The listing builds one solid part. Answer for the finished solid, in the listing's coordinates (mm). Face numbers are marked on the shaded views. Coordinates: 2 decimals unless noted, no trailing zeros. Order: outer loops, then holes, each group sorted by start corner. A loop starts at its lowest first (then second) coordinate and runs counter-clockwise, first axis right, second up. Notation, with made-up numbers: M 10,30.25 L 31,30.25 A15 ccw 31,45.25 Z; hole C 52,59.5 d9. An arc over 180 degrees is marked long. One line per item, written item: value. Start each with the question number.
Q1. Each of these flat-tipped pins is pushed along its axis until it touches: pin 1 Ø5 at (x, z) = (-2, 1) entering from -Y; pin 2 Ø2 at (x, y) = (3, 2) entering from -Z; pin 3 Ø4 at (x, z) = (-3.5, 3.5) entering from +Y; pin 4 Ø5 at (x, y) = (3, -3.5) entering from -Z. Where does it stop, or does it pass through?
Q2. Straight lines are drawn through the part: line 1 along Z through (x, y) = (0, -2); line 2 along X through (y, z) = (1.25, 2); line 3 along X through (y, z) = (-1, -0.5). For each, find the intervals that lie inside material, in ascending order. Write a range as [from, to].
Q3. The part is cut by section B-B on z = 0. Give the vertices of the cut face in (x, y), then the cut area to 3 significant figures.
Q4. Determine the mould class of the marked faces 1 and 2 for opening direction Z: pulls with the +Z half, pulls with the -Z half, needs draft (parallel to the pull), parting line crosses it, or undercut.
Q5. The part is cut by section A-A on x = 0. Give the vertices of the cut face in (y, z).
Q6. The part is cut by section C-C on y = 4. Give the vertices of the cut face in (x, z).
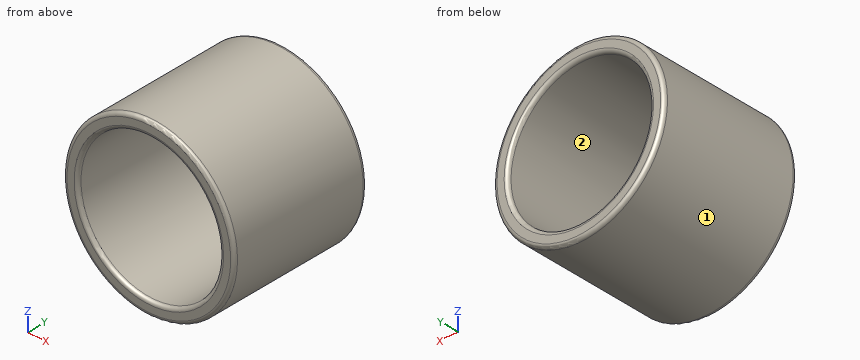
```python
from build123d import *

# Parameters (mm, degrees)
F0_R     = 6
F0_R_2   = 5
F1_DEPTH = 5
F2_R     = 0.25


with BuildPart() as f1:
    # F0 (on Front) → F1 (new body, symmetric)
    with BuildSketch(Plane.XZ):
        Circle(F0_R)
        Circle(F0_R_2, mode=Mode.SUBTRACT)
    extrude(amount=F1_DEPTH, both=True)

    # F2
    f2_edges = [f1.edges().sort_by_distance(p)[0] for p in [
        (-6, -5, 0),
        (-5, -5, 0),
        (-6, 5, 0),
        (-5, 5, 0),
    ]]
    fillet(f2_edges, radius=F2_R)


solid = f1.part
```
Output:
1. pin 1: passes through
1. pin 2: stops at z = -5.66
1. pin 3: stops at y = 5
1. pin 4: stops at z = -5.98
2. line 1: z = [-6, -5], [5, 6]
2. line 2: x = [-5.66, -4.58], [4.58, 5.66]
2. line 3: x = [-5.98, -4.97], [4.97, 5.98]
3. outline: M -6,-4.75 A0.25 ccw -5.75,-5 L -5.25,-5 A0.25 ccw -5,-4.75 L -5,4.75 A0.25 ccw -5.25,5 L -5.75,5 A0.25 ccw -6,4.75 Z; M 5,-4.75 A0.25 ccw 5.25,-5 L 5.75,-5 A0.25 ccw 6,-4.75 L 6,4.75 A0.25 ccw 5.75,5 L 5.25,5 A0.25 ccw 5,4.75 Z
3. area: 19.9 mm^2
4. face 1: parting line crosses it
4. face 2: undercut
5. outline: M -5,-5.75 A0.25 ccw -4.75,-6 L 4.75,-6 A0.25 ccw 5,-5.75 L 5,-5.25 A0.25 ccw 4.75,-5 L -4.75,-5 A0.25 ccw -5,-5.25 Z; M -5,5.25 A0.25 ccw -4.75,5 L 4.75,5 A0.25 ccw 5,5.25 L 5,5.75 A0.25 ccw 4.75,6 L -4.75,6 A0.25 ccw -5,5.75 Z
6. outline: C 0,0 d12; hole C 0,0 d10
